Here's how the part is built. I have some questions about the finished solid (model axes, mm). Face numbers are marked on the shaded views. Coordinates: 2 decimals unless noted, no trailing zeros. Loops run counter-clockwise (first coordinate to the right, second up) from the corner with the lowest first, then second, coordinate; pieces in that order, holes last. Notation, with made-up numbers: (2.5, 18) -> (20.5, 18) arc R29 cw to (20.5, 45) -> close; hole circle Ø2 at (51.25, 56.5). An arc over 180 degrees is marked (long way). Answer as a JSON object with one key per item and string values. Group by question number.
1) I need wall thicknesses on probe 1 along X at (y, z) = (29, 9); probe 2 along Y at (x, z) = (46, 19); probe 3 along Y at (x, z) = (50, 2.3). Which ranges of each line are inside material? Lowest first, please. Write a range as [from, to].
2) I'm going to push flat-ended pins straight in: pin 1 (6 mm diameter, centred on x = 78.5, y = 35.5, fed in from +Z); pin 2 (7.5 mm diameter, centred on x = 59.36, z = 16.98, fed in from +Y). Where does each tip first touch, or does it pass through?
3) If we mould it in two halves opening along Y, with no side actions, what happens to the marked faces 1, 2 and 3? For each: +Y half, -Y half, draft (parallel to the pull), parting line (faces both ways), or undercut.
4) I want a section at B-B (y = 23). Write out the boundary of the cut face in (x, z), then the cut area to 3 significant figures.
5) I want a section at D-D (x = 88). Count the separate pieces of the cut face and the enclosed holes in it, then the cut area to 3 significant figures.
6) I want a section at A-A (x = 50). Write out the boundary of the cut face in (y, z) (3 decimals), then the cut area to 3 significant figures.
7) I want a section at C-C (y = 34.5). Write out the boundary of the cut face in (x, z).
```python
from build123d import *

# Parameters (mm, degrees)
SKETCH_W          = 100
SKETCH_H          = 45
PAD_DEPTH         = 20
PAD_FACE2_W       = 45
PAD_FACE2_H       = 20
POCKET_DEPTH      = 3
POCKET_FACE5_W    = 45
POCKET_FACE5_H    = 20
POCKET001_DEPTH   = 3
POCKET001_FACE1_W = 94
POCKET001_FACE1_H = 20
POCKET002_DEPTH   = 8
POCKET003_DEPTH   = 20
POCKET004_DEPTH   = 17
PAD001_DEPTH      = 2
SKETCH003_R       = 4.025
POCKET005_DEPTH   = 5
SKETCH004_R       = 4.025
POCKET006_DEPTH   = 5
SKETCH005_R       = 4.025
POCKET007_DEPTH   = 5
SKETCH006_R       = 4
SKETCH006_R_2     = 2
POCKET008_DEPTH   = 5
SKETCH007_R       = 3
POCKET009_DEPTH   = 1
PAD002_DEPTH      = 1
SKETCH008_R       = 4.05
POCKET010_DEPTH   = 5
SKETCH009_R       = 4.05
POCKET011_DEPTH   = 5
SKETCH010_R       = 4.05
POCKET012_DEPTH   = 5
SKETCH011_R       = 4
POCKET013_DEPTH   = 5
SKETCH012_W       = 15.333549
SKETCH012_H       = 10.93085
PAD003_DEPTH      = 3


with BuildPart() as part:
    # Sketch → Pad (new body)
    with BuildSketch(Plane.XY):
        with Locations((50, 22.5)):
            Rectangle(SKETCH_W, SKETCH_H)
    extrude(amount=PAD_DEPTH)

    # Pad Face2 → Pocket (cut)
    with BuildSketch(Plane(origin=(100, 22.5, 10), x_dir=(0, -1, 0), z_dir=(1, 0, 0))):
        Rectangle(PAD_FACE2_W, PAD_FACE2_H)
    extrude(amount=-POCKET_DEPTH, mode=Mode.SUBTRACT)

    # Pocket Face5 → Pocket001 (cut)
    with BuildSketch(Plane(origin=(0, 22.5, 10), x_dir=(0, 1, 0), z_dir=(-1, 0, 0))):
        Rectangle(POCKET_FACE5_W, POCKET_FACE5_H)
    extrude(amount=-POCKET001_DEPTH, mode=Mode.SUBTRACT)

    # Pocket001 Face1 → Pocket002 (cut)
    with BuildSketch(Plane(origin=(50, 0, 10), x_dir=(-1, 0, 0), z_dir=(0, -1, 0))):
        Rectangle(POCKET001_FACE1_W, POCKET001_FACE1_H)
    extrude(amount=-POCKET002_DEPTH, mode=Mode.SUBTRACT)

    # Sketch001 (on Face6 of Pocket002) → Pocket003 (cut)
    with BuildSketch(Plane.XY.offset(20)):
        Polygon((3, 45), (3, 39.13), (35.3, 45), align=None)
        Polygon((64.7, 45), (97, 45), (97, 39.13), align=None)
    extrude(amount=-POCKET003_DEPTH, mode=Mode.SUBTRACT)

    # Sketch002 (on Face8 of Pocket003) → Pocket004 (cut)
    with BuildSketch(Plane.XY.offset(20)):
        Polygon((6, 36.6260629355), (6, 11), (94, 11), (94, 36.6260629355), (64.6580556127, 42), (35.3419443873, 42), align=None)
    extrude(amount=-POCKET004_DEPTH, mode=Mode.SUBTRACT)

    # Pocket004 Face8 → Pad001 (add)
    with BuildSketch(Plane(origin=(50, 25.1421826555, 20), x_dir=(0, 1, 0), z_dir=(0, 0, 1))):
        Polygon((-17.1421826555, 47), (-17.1421826555, -47), (13.9878173445, -47), (19.8578173445, -14.7), (19.8578173445, 14.7), (13.9878173445, 47), align=None)
        Polygon((-14.1421826555, 44), (11.4838802799, 44), (16.8578173445, 14.6580556127), (16.8578173445, -14.6580556127), (11.4838802799, -44), (-14.1421826555, -44), align=None, mode=Mode.SUBTRACT)
    extrude(amount=PAD001_DEPTH)

    # Sketch003 (on Face6 of Pad001) → Pocket005 (cut)
    with BuildSketch(Plane(origin=(0, 45, 0), x_dir=(-1, 0, 0), z_dir=(0, 1, 0))):
        with Locations((-59.3625, 16.975)):
            Circle(SKETCH003_R)
        with Locations((-50, 16.975)):
            Circle(SKETCH003_R)
        with Locations((-40.6375, 16.975)):
            Circle(SKETCH003_R)
        with Locations((-59.3625, 7.525)):
            Circle(SKETCH003_R)
        with Locations((-50, 7.525)):
            Circle(SKETCH003_R)
        with Locations((-40.6375, 7.525)):
            Circle(SKETCH003_R)
    extrude(amount=-POCKET005_DEPTH, mode=Mode.SUBTRACT)

    # Sketch004 (on Face6 of Pocket005) → Pocket006 (cut)
    with BuildSketch(Plane(origin=(9.9850961575, 54.9435444444, 0), x_dir=(-0.983884528, 0.178805021, 0), z_dir=(0.178805021, 0.983884528, 0))):
        with Locations((-80.0098530156, 16.975)):
            Circle(SKETCH004_R)
        with Locations((-70.9736030156, 16.975)):
            Circle(SKETCH004_R)
        with Locations((-61.6111030156, 16.975)):
            Circle(SKETCH004_R)
        with Locations((-80.3361030156, 7.525)):
            Circle(SKETCH004_R)
        with Locations((-70.9736030156, 7.525)):
            Circle(SKETCH004_R)
        with Locations((-61.6111030156, 7.525)):
            Circle(SKETCH004_R)
    extrude(amount=-POCKET006_DEPTH, mode=Mode.SUBTRACT)

    # Sketch005 (on Face4 of Pocket006) → Pocket007 (cut)
    with BuildSketch(Plane(origin=(-6.7879726028, 37.3511950719, 0), x_dir=(-0.983884528, -0.178805021, 0), z_dir=(-0.178805021, 0.983884528, 0))):
        with Locations((-36.7773497852, 16.975)):
            Circle(SKETCH005_R)
        with Locations((-27.4148497852, 16.975)):
            Circle(SKETCH005_R)
        with Locations((-18.0523497852, 16.975)):
            Circle(SKETCH005_R)
        with Locations((-36.7773497852, 7.525)):
            Circle(SKETCH005_R)
        with Locations((-27.4148497852, 7.525)):
            Circle(SKETCH005_R)
        with Locations((-18.0523497852, 7.525)):
            Circle(SKETCH005_R)
    extrude(amount=-POCKET007_DEPTH, mode=Mode.SUBTRACT)

    # Sketch006 (on Face1 of Pocket007) → Pocket008 (cut)
    with BuildSketch(Plane(origin=(0, 0, 0), x_dir=(1, 0, 0), z_dir=(0, 0, -1))):
        with Locations((50, -23)):
            Circle(SKETCH006_R)
        with Locations((65.7, -18)):
            Circle(SKETCH006_R_2)
        with Locations((34.3, -18)):
            Circle(SKETCH006_R_2)
        with Locations((20, -23)):
            Circle(SKETCH006_R_2)
        with Locations((80, -23)):
            Circle(SKETCH006_R_2)
    extrude(amount=-POCKET008_DEPTH, mode=Mode.SUBTRACT)

    # Sketch007 (on Face1 of Pocket008) → Pocket009 (cut)
    with BuildSketch(Plane(origin=(0, 0, 0), x_dir=(1, 0, 0), z_dir=(0, 0, -1))):
        with Locations((20, -23)):
            Circle(SKETCH007_R)
        with Locations((80, -23)):
            Circle(SKETCH007_R)
    extrude(amount=-POCKET009_DEPTH, mode=Mode.SUBTRACT)

    # Pocket009 Face13 → Pad002 (add)
    with BuildSketch(Plane(origin=(50, 25.1421826555, 22), x_dir=(0, 1, 0), z_dir=(0, 0, 1))):
        Polygon((-17.1421826555, 47), (-17.1421826555, -47), (13.9878173445, -47), (19.8578173445, -14.7), (19.8578173445, 14.7), (13.9878173445, 47), align=None)
        Polygon((-14.1421826555, 44), (11.4838802799, 44), (16.8578173445, 14.6580556127), (16.8578173445, -14.6580556127), (11.4838802799, -44), (-14.1421826555, -44), align=None, mode=Mode.SUBTRACT)
    extrude(amount=PAD002_DEPTH)

    # Sketch008 (on Face30 of Pad002) → Pocket010 (cut)
    with BuildSketch(Plane(origin=(0, 45, 0), x_dir=(-1, 0, 0), z_dir=(0, 1, 0))):
        with Locations((-59.3625, 16.975)):
            Circle(SKETCH008_R)
        with Locations((-50.000011, 16.975002)):
            Circle(SKETCH008_R)
        with Locations((-40.6375, 16.975)):
            Circle(SKETCH008_R)
        with Locations((-40.6375, 7.525)):
            Circle(SKETCH008_R)
        with Locations((-50, 7.525)):
            Circle(SKETCH008_R)
        with Locations((-59.3625, 7.525)):
            Circle(SKETCH008_R)
    extrude(amount=-POCKET010_DEPTH, mode=Mode.SUBTRACT)

    # Sketch009 (on Face6 of Pocket010) → Pocket011 (cut)
    with BuildSketch(Plane(origin=(9.9850961575, 54.9435444444, 0), x_dir=(-0.983884528, 0.178805021, 0), z_dir=(0.178805021, 0.983884528, 0))):
        with Locations((-80.0098530156, 16.975)):
            Circle(SKETCH009_R)
        with Locations((-70.9736030156, 16.975)):
            Circle(SKETCH009_R)
        with Locations((-61.6111030156, 16.975)):
            Circle(SKETCH009_R)
        with Locations((-61.6111030156, 7.525)):
            Circle(SKETCH009_R)
        with Locations((-70.9736030156, 7.525)):
            Circle(SKETCH009_R)
        with Locations((-80.3361030156, 7.525)):
            Circle(SKETCH009_R)
    extrude(amount=-POCKET011_DEPTH, mode=Mode.SUBTRACT)

    # Sketch010 (on Face5 of Pocket011) → Pocket012 (cut)
    with BuildSketch(Plane(origin=(-6.7879726028, 37.3511950719, 0), x_dir=(-0.983884528, -0.178805021, 0), z_dir=(-0.178805021, 0.983884528, 0))):
        with Locations((-36.7773497852, 16.975)):
            Circle(SKETCH010_R)
        with Locations((-27.4148497852, 16.975)):
            Circle(SKETCH010_R)
        with Locations((-18.0523497852, 16.975)):
            Circle(SKETCH010_R)
        with Locations((-18.0523497852, 7.525)):
            Circle(SKETCH010_R)
        with Locations((-27.4148497852, 7.525)):
            Circle(SKETCH010_R)
        with Locations((-36.7773497852, 7.525)):
            Circle(SKETCH010_R)
    extrude(amount=-POCKET012_DEPTH, mode=Mode.SUBTRACT)

    # Sketch011 (on Face3 of Pocket012) → Pocket013 (cut)
    with BuildSketch(Plane(origin=(3, 0, 0), x_dir=(0, -1, 0), z_dir=(-1, 0, 0))):
        with Locations((-20, 15)):
            Circle(SKETCH011_R)
    extrude(amount=-POCKET013_DEPTH, mode=Mode.SUBTRACT)

    # Sketch012 (on Face3 of Pocket013) → Pad003 (join)
    with BuildSketch(Plane(origin=(3, 0, 0), x_dir=(0, -1, 0), z_dir=(-1, 0, 0))):
        with Locations((-20.0389255, 14.391196)):
            Rectangle(SKETCH012_W, SKETCH012_H)
    extrude(amount=-PAD003_DEPTH)


solid = part.part
```
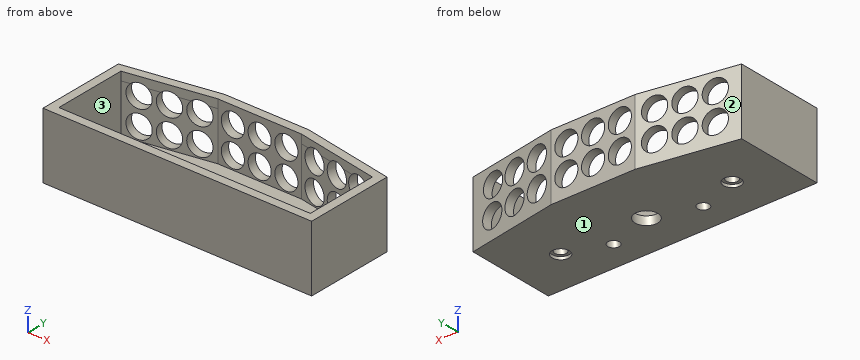
Determined:
{
 "1": {"probe 1": "[3, 6], [94, 97]", "probe 2": "[8, 11], [42, 45]", "probe 3": "[8, 19], [27, 45]"},
 "2": {"pin 1": "z = 3", "pin 2": "y = 11"},
 "3": {"face 1": "draft", "face 2": "+Y half", "face 3": "undercut"},
 "4": {"outline": "(3, 0) -> (17, 0) -> (17, 1) -> (18, 1) -> (18, 3) -> (6, 3) -> (6, 23) -> (3, 23) -> close; (22, 1) -> (23, 1) -> (23, 0) -> (46, 0) -> (46, 3) -> (22, 3) -> close; (54, 0) -> (77, 0) -> (77, 1) -> (78, 1) -> (78, 3) -> (54, 3) -> close; (82, 1) -> (83, 1) -> (83, 0) -> (97, 0) -> (97, 23) -> (94, 23) -> (94, 3) -> (82, 3) -> close", "area": "350 mm^2"},
 "5": {"separate pieces": "3", "enclosed holes": "0", "area": "170 mm^2"},
 "6": {"outline": "(8, 0) -> (19, 0) -> (19, 3) -> (11, 3) -> (11, 23) -> (8, 23) -> close; (27, 0) -> (45, 0) -> (45, 3.475) -> (42, 3.475) -> (42, 3) -> (27, 3) -> close; (42, 11.575) -> (45, 11.575) -> (45, 12.925) -> (42, 12.925) -> close; (42, 21.025) -> (45, 21.025) -> (45, 23) -> (42, 23) -> close", "area": "158 mm^2"},
 "7": {"outline": "(3, 0) -> (97, 0) -> (97, 23) -> (94, 23) -> (94, 3) -> (6, 3) -> (6, 23) -> (3, 23) -> close"}
}
